Geometry: final body of the model. Coordinates: model frame, mm. A direction names the side the tool comes from. Round coordinates to 2 decimals unless told otherwise and drop trailing zeros. Loops run counter-clockwise (first coordinate to the right, second up) from the corner with the lowest first, then second, coordinate; pieces in that order, holes last. Notation, with made-up numbers: (-6, 78) - (35, 78) arc R20 ccw to (35, 97) - close; hole circle Ø2 at (-22, 42). An arc over 180 degrees is marked (long way). Return JSON: item names as keys, results as strings. Group by question number.
1. First-contact query: pin 1 Ø4 at (y, z) = (7.6, 10) entering from +X; pin 2 Ø4 at (x, z) = (2.5, 74.5) entering from +Y; pin 3 Ø2.5 at (x, z) = (2.5, 77.5) entering from -Y. Flat tips, straight axial feed; report the tip coordinate or a pass-through.
2. Section D-D on z = 48.5. Return loops of the section in (x, y).
3. Draft query along Y for faces 4 (the face through (-1.5, 6, 110.6)), 5 (the face through (3, 0.1, 61)), 6 (the face through (-2, 18.2, 60)). Return one class per face: +Y half, -Y half, draft (parallel to the pull), parting line (faces both ways), or undercut.
4. Section B-B on y = 7.6. Count the separate pieces of the cut face and the enclosed holes in it, and give its area (3 significant figures).
5. Section A-A on z = 111. Return loops of the section in (x, y), and give its area (3 significant figures).
6. Material intervals for probe 1 along Y at (x, z) = (-0.6, 10); probe 2 along Z at (x, y) = (-2.5, 8.75); probe 3 along Z at (x, y) = (-0.5, 8.5), sorted ascending.
7. Set-up query: faces 1 (the face through (3, 15.1, 61)), 2 (the face through (0, -2, 75)), 3 (the face through (-1.5, 6, 9.6)). Return all of +Z, -Z, +X, -X, +Y, -Y with unobstructed straight access to the full face (end or side cutting, diameter ignored); none if empty.
from build123d import *

# Parameters (mm, degrees)
SKETCH_1_W          = 21.2
SKETCH_1_H          = 21.2
SKETCH_1_W_2        = 15.2
SKETCH_1_H_2        = 15.2
EXTRUDE_1_DEPTH     = 121
SKETCH_2_R          = 1.65
CUT_EXTRUDE_1_DEPTH = 30
SKETCH_3_W          = 121
SKETCH_3_H          = 21.2
CUT_EXTRUDE_2_DEPTH = 18.2
SKETCH_4_W          = 68.8
SKETCH_4_H          = 15
EXTRUDE_1_2_DEPTH   = 5.1
CHAMFER_1_SIZE      = 5.1


with BuildPart() as part:
    # 草图1 → Extrude 1 (new body)
    with BuildSketch(Plane.XY):
        with Locations((7.6, 7.6)):
            Rectangle(SKETCH_1_W, SKETCH_1_H)
        with Locations((7.6, 7.6)):
            Rectangle(SKETCH_1_W_2, SKETCH_1_H_2, mode=Mode.SUBTRACT)
    extrude(amount=EXTRUDE_1_DEPTH)

    # 草图2 → 切除-拉伸1 (cut)
    with BuildSketch(Plane.ZY.offset(3)):
        with Locations((10, 7.6)):
            Circle(SKETCH_2_R)
        with Locations((111, 7.6)):
            Circle(SKETCH_2_R)
    extrude(amount=-CUT_EXTRUDE_1_DEPTH, mode=Mode.SUBTRACT)

    # 草图3 → 切除-拉伸2 (cut)
    with BuildSketch(Plane(origin=(18.2, 0, 0), x_dir=(0, 0, -1), z_dir=(1, 0, 0))):
        with Locations((-60.5, 7.6)):
            Rectangle(SKETCH_3_W, SKETCH_3_H)
    extrude(amount=-CUT_EXTRUDE_2_DEPTH, mode=Mode.SUBTRACT)

    # 草图4 → Extrude 1 2 (add)
    with BuildSketch(Plane(origin=(0, 0, 0), x_dir=(0, 0, -1), z_dir=(1, 0, 0))):
        with Locations((-60.5, 7.6)):
            Rectangle(SKETCH_4_W, SKETCH_4_H)
    extrude(amount=EXTRUDE_1_2_DEPTH)

    # 倒角1
    chamfer_1_edges = [part.edges().sort_by_distance(p)[0] for p in [
        (0, 7.6, 26.1),
        (0, 7.6, 94.9),
    ]]
    chamfer(chamfer_1_edges, length=CHAMFER_1_SIZE - 0.0001)  # a hair under: the kernel refuses the full size


solid = part.part
Taken from the geometry:
{
 "1": {"pin 1": "x = 0", "pin 2": "y = 15.1", "pin 3": "y = 0.1"},
 "2": {"outline": "(-3, -3) - (0, -3) - (0, 0.1) - (5.1, 0.1) - (5.1, 15.1) - (0, 15.1) - (0, 18.2) - (-3, 18.2) - close"},
 "3": {"face 4": "undercut", "face 5": "-Y half", "face 6": "+Y half"},
 "4": {"separate pieces": "3", "enclosed holes": "0", "area": "720 mm2"},
 "5": {"outline": "(-3, -3) - (0, -3) - (0, 5.95) - (-3, 5.95) - close; (-3, 9.25) - (0, 9.25) - (0, 18.2) - (-3, 18.2) - close", "area": "53.7 mm2"},
 "6": {"probe 1": "-3 to 5.95, 9.25 to 18.2", "probe 2": "0 to 8.82, 11.18 to 109.82, 112.18 to 121", "probe 3": "0 to 8.62, 11.38 to 109.62, 112.38 to 121"},
 "7": {"face 1": "+Z, -Z, +X, +Y", "face 2": "+X", "face 3": "+X, -X"}
}
